from build123d import *

# Parameters (mm, degrees)
SKETCH_W  = 130
SKETCH_H  = 40
SKETCH_R  = 1.5625
PAD_DEPTH = 2.5
FILLET_R  = 3


with BuildPart() as part:
    # Sketch → Pad (new body)
    with BuildSketch(Plane.XY):
        with Locations((65, 20)):
            Rectangle(SKETCH_W, SKETCH_H)
        with Locations((20, 25)):
            Circle(SKETCH_R, mode=Mode.SUBTRACT)
        with Locations((40, 25)):
            Circle(SKETCH_R, mode=Mode.SUBTRACT)
        with Locations((30, 15)):
            Circle(SKETCH_R, mode=Mode.SUBTRACT)
        with Locations((50, 15)):
            Circle(SKETCH_R, mode=Mode.SUBTRACT)
        with Locations((110, 25)):
            Circle(SKETCH_R, mode=Mode.SUBTRACT)
        with Locations((90, 25)):
            Circle(SKETCH_R, mode=Mode.SUBTRACT)
        with Locations((100, 15)):
            Circle(SKETCH_R, mode=Mode.SUBTRACT)
        with Locations((80, 15)):
            Circle(SKETCH_R, mode=Mode.SUBTRACT)
    extrude(amount=PAD_DEPTH)

    # Fillet
    fillet_edges = [part.edges().sort_by_distance(p)[0] for p in [
        (0, 0, 1.25),
        (130, 0, 1.25),
        (130, 40, 1.25),
        (0, 40, 1.25),
    ]]
    fillet(fillet_edges, radius=FILLET_R)


solid = part.part
Could you check a few things on this model? Use its own coordinates, in mm. Give positions to 0.01 mm unless a question says otherwise; leave off trailing zeros. Write each loop counter-clockwise with the first axis right and the second up, starting at its lowest first coordinate (ties: lowest second). Pieces come first, ordered by that corner, then holes. Notation, with made-up numbers: (48, 2) -> (89, 2) arc R23 ccw to (89, 32) -> close; hole circle Ø11 at (89, 16). An arc over 180 degrees is marked (long way). Answer as CSV lines item,"result". Start each with the question number.
(1) If we section it at B-B, the plane x = 20: Write out the boundary of the cut face in (y, z), and give its area (3 significant figures).
(2) If we mould it in two halves opening along Y, with no side actions, what happens to faces 1 (the face through (78.85, 16.06, 1.23)), 2 (the face through (0.86, 0.9, 1.27)), 3 (the face through (130, 20, 1))? For each: +Y half, -Y half, draft (parallel to the pull), parting line (faces both ways), or undercut.
(3) If we section it at A-A, the plane y = 25: Write out the boundary of the cut face in (x, z).
(4) Please list where these lines run through material, in increasing order: line 1 (X direction, y = 14.5, z = 2.3); line 2 (Y direction, x = 80, z = 1.75); line 3 (Y direction, x = 29, z = 1.75).
Answer list:
1,outline,"(0, 0) -> (23.44, 0) -> (23.44, 2.5) -> (0, 2.5) -> close; (26.56, 0) -> (40, 0) -> (40, 2.5) -> (26.56, 2.5) -> close"
1,area,"92.2 mm^2"
2,face 1,"undercut"
2,face 2,"-Y half"
2,face 3,"draft"
3,outline,"(0, 0) -> (18.44, 0) -> (18.44, 2.5) -> (0, 2.5) -> close; (21.56, 0) -> (38.44, 0) -> (38.44, 2.5) -> (21.56, 2.5) -> close; (41.56, 0) -> (88.44, 0) -> (88.44, 2.5) -> (41.56, 2.5) -> close; (91.56, 0) -> (108.44, 0) -> (108.44, 2.5) -> (91.56, 2.5) -> close; (111.56, 0) -> (130, 0) -> (130, 2.5) -> (111.56, 2.5) -> close"
4,line 1,"0 to 28.52, 31.48 to 48.52, 51.48 to 78.52, 81.48 to 98.52, 101.48 to 130"
4,line 2,"0 to 13.44, 16.56 to 40"
4,line 3,"0 to 13.8, 16.2 to 40"
